```python
from build123d import *

# Parameters (mm, degrees)
F0_W     = 60.96
F0_H     = 104.14
F0_W_2   = 49.7204400599
F0_H_2   = 36.4855006337
F1_DEPTH = 10.414
F2_W     = 25.4
F2_H     = 1.27
F3_DEPTH = 10.16
F4_R     = 1.8844419378
F5_DEPTH = 19.05
F6_W     = 11.8811856955
F6_H     = 2.1055263933
F7_DEPTH = 2.54
F8_R     = 0.762


with BuildPart() as f1:
    # F0 (on Top) → F1 (new body)
    with BuildSketch(Plane.XY):
        Rectangle(F0_W, F0_H)
        with Locations((-0.3395788372, 28.8962163031)):
            Rectangle(F0_W_2, F0_H_2, mode=Mode.SUBTRACT)
        with Locations((-0.3395788372, 28.8962163031)):
            Rectangle(F0_W_2, F0_H_2)
    extrude(amount=F1_DEPTH)

    # F2 (on face) → F3 (cut)
    with BuildSketch(Plane.XZ.offset(52.07)):
        with Locations((0, 4.7498)):
            Rectangle(F2_W, F2_H)
    extrude(amount=-F3_DEPTH, mode=Mode.SUBTRACT)

    # F4 (on face) → F5 (cut)
    with BuildSketch(Plane(origin=(0, 52.07, 0), x_dir=(-1, 0, 0), z_dir=(0, 1, 0))):
        with Locations((24.78357777, 4.7017154284)):
            Circle(F4_R)
    extrude(amount=-F5_DEPTH, mode=Mode.SUBTRACT)

    # F6 (on face) → F7 (join)
    with BuildSketch(Plane(origin=(0, 52.07, 0), x_dir=(-1, 0, 0), z_dir=(0, 1, 0))):
        with Locations((-19.3572798744, 4.8521101708)):
            Rectangle(F6_W, F6_H)
    extrude(amount=F7_DEPTH)

    # F8
    f8_edges = [f1.edges().sort_by_distance(p)[0] for p in [
        (13.416687, 53.34, 3.799347),
        (25.297873, 53.34, 3.799347),
        (25.297873, 53.34, 5.904873),
        (13.416687, 53.34, 5.904873),
    ]]
    fillet(f8_edges, radius=F8_R)


solid = f1.part
```
Part model, mm, in its own coordinate system. A direction names the side the tool comes from. Round coordinates to 2 decimals unless told otherwise and drop trailing zeros. Order: outer loops, then holes, each group sorted by start corner. A loop starts at its lowest first (then second) coordinate and runs counter-clockwise, first axis right, second up. Notation, with made-up numbers: M 63,-3.5 L 95,-3.5 A11 ccw 95,1.5 Z; hole C 23,-33.5 d6. An arc over 180 degrees is marked long. Put each result on its own line as item: value. Start each with the question number.
1. Drop flat-ended pins along their axis: pin 1 (0.6 mm diameter, centred on x = 2.5, z = 4.5, fed in from -Y); pin 2 (1.3 mm diameter, centred on x = 17.5, y = 53, fed in from +Z); pin 3 (3 mm diameter, centred on x = 20, y = 52.5, fed in from -Z); pin 4 (4 mm diameter, centred on x = -24.5, z = 5, fed in from +Y). Give the stop position or say it passes through.
2. Drill centre lines: probe 1 along Y at (x, z) = (-23, 1.5); probe 2 along X at (y, z) = (39.5, 5); probe 3 along Z at (x, y) = (-24, 37). Where is each one in solid material? Low to high. Write a range as [from, to].
3. Two-plate mould, pull along X, no slides. Class faces 1 (the face through (-25, 33.02, 5)), 2 (the face through (-30.48, -1, 5)), 3 (the face through (19, 53, 5.905)): +X half, -X half, draft (parallel to the pull), parting line (faces both ways), or undercut.
4. Slice it at A-A on x = 22.5. List the corners of the cut face in (y, z), then the cut area to 3 significant figures.
5. Slice it at D-D on z = 1.75. List the corners of the cut face in (x, y).
6. Slice it at B-B on y = 41. List the corners of the cut face in (x, z), then the cut area to 3 significant figures.
7. Tool access for faces 4 (the face through (19, 53, 3.799)), 5 (the face through (-25.65, 42.68, 3.03)), 6 (the face through (30.48, -1, 5)), 7 (the face through (0, -47, 5.385)), 8 (the face through (0, -52.07, 6)): list every direction of +Z, -Z, +X, -X, +Y, -Y with a clear straight run to the whole face (end or side of a thin tool).
8. Slice it at C-C on x = -1.5. List the corners of the cut face in (y, z), then the cut area to 3 significant figures.
Findings:
1. pin 1: y = -41.91
1. pin 2: z = 5.9
1. pin 3: z = 0
1. pin 4: y = 52.07
2. probe 1: [-52.07, 52.07]
2. probe 2: [-30.48, -26.64], [-22.92, 30.48]
2. probe 3: [0, 2.99], [6.42, 10.41]
3. face 1: undercut
3. face 2: -X half
3. face 3: draft
4. outline: M -52.07,0 L 52.07,0 L 52.07,3.8 L 54.61,3.8 L 54.61,5.9 L 52.07,5.9 L 52.07,10.41 L -52.07,10.41 Z
4. area: 1,090 mm2
5. outline: M -30.48,-52.07 L 30.48,-52.07 L 30.48,52.07 L -30.48,52.07 Z
6. outline: M -30.48,0 L 30.48,0 L 30.48,10.41 L -30.48,10.41 Z; hole C -24.78,4.7 d3.77
6. area: 624 mm2
7. face 4: -Z, +X, -X, +Y
7. face 5: +Y
7. face 6: +Z, -Z, +X, +Y, -Y
7. face 7: -Y
7. face 8: +Z, -Z, +X, -X, -Y
8. outline: M -52.07,0 L 52.07,0 L 52.07,10.41 L -52.07,10.41 L -52.07,5.38 L -41.91,5.38 L -41.91,4.11 L -52.07,4.11 Z
8. area: 1,070 mm2
